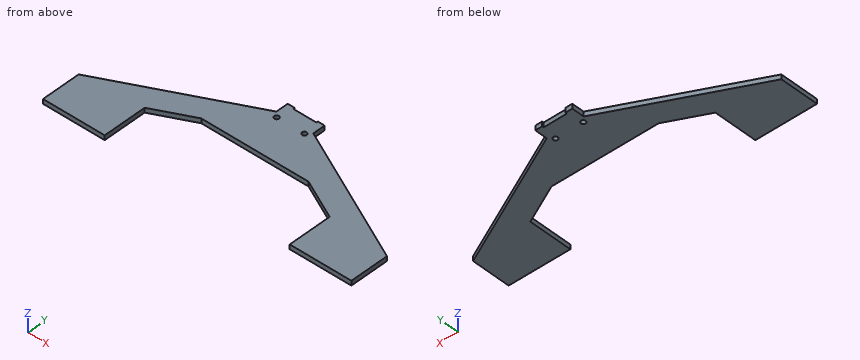
from build123d import *

# Parameters (mm, degrees)
EXTRUDE_1_DEPTH     = 3
SKETCH_3_R          = 1.5
CUT_EXTRUDE_1_DEPTH = 3


with BuildPart() as part:
    # 草图2 → 凸台-拉伸1 (new body)
    with BuildSketch(Plane(origin=(356.17996861, -2895.528235046, -3033.98121825), x_dir=(1, 0, 0), z_dir=(0, 0, 1))):
        Polygon((-296.17996861, 2848.06839364), (-321.386084558, 2860.528235046), (-390.973852662, 2860.528235046), (-416.17996861, 2848.06839364), (-416.17996861, 2820.028235046), (-456.17996861, 2820.028235046), (-456.17996861, 2845.028235046), (-368.17996861, 2888.528235046), (-368.17996861, 2896.528235046), (-363.67996861, 2896.528235046), (-363.67996861, 2895.528235046), (-348.67996861, 2895.528235046), (-348.67996861, 2896.528235046), (-344.17996861, 2896.528235046), (-344.17996861, 2888.528235046), (-256.17996861, 2845.028235046), (-256.17996861, 2820.028235046), (-296.17996861, 2820.028235046), align=None)
    extrude(amount=EXTRUDE_1_DEPTH)

    # 草图3 → 切除-拉伸1 (cut)
    with BuildSketch(Plane.XY.offset(-3030.98121825)):
        with Locations((9, -10)):
            Circle(SKETCH_3_R)
        with Locations((-9, -10)):
            Circle(SKETCH_3_R)
    extrude(amount=-CUT_EXTRUDE_1_DEPTH, mode=Mode.SUBTRACT)


solid = part.part
Input: part model. Units: mm. Frame: model coordinates. Round coordinates to 2 decimals unless told otherwise and drop trailing zeros. Loops run counter-clockwise (first coordinate to the right, second up) from the corner with the lowest first, then second, coordinate; pieces in that order, holes last. Notation, with made-up numbers: (65, -38) -> (84, -38) arc R16 ccw to (84, -11) -> close; hole circle Ø5 at (-23.75, 57). An arc over 180 degrees is marked (long way). Answer as a JSON object with one key per item and string values. Group by question number.
1) Section query D-D on x = -51.5. Output: boundary loops of the cut face in (y, z), plus the area to 3 significant figures.
2) Section query C-C on y = -30. Output: boundary loops of the cut face in (x, z).
3) Section query A-A on z = -3031.7. Output: boundary loops of the cut face in (x, y).
4) Ray query, L1, parallel to X at y = -52, z = -3032.15; L2, parallel to Y at x = -9, z = -3031.8; L3, parallel to Y at x = 5.5, z = -3032.4. Return the intervals inside material, ascending.
5) Pin query (flat end, axial travel): pin 1 (0.9 mm diameter, centred on x = -2.5, z = -3032, fed in from +Y). Return the tip coordinate at first contact, or that it passes through.
6) Section query B-B on y = -69. Output: boundary loops of the cut face in (x, z), plus the area to 3 significant figures.
Reply:
{
 "1": {"outline": "(-43.26, -3033.98) -> (-26.53, -3033.98) -> (-26.53, -3030.98) -> (-43.26, -3030.98) -> close", "area": "50.2 mm2"},
 "2": {"outline": "(-58.53, -3033.98) -> (58.53, -3033.98) -> (58.53, -3030.98) -> (-58.53, -3030.98) -> close"},
 "3": {"outline": "(-100, -75.5) -> (-60, -75.5) -> (-60, -47.46) -> (-34.79, -35) -> (34.79, -35) -> (60, -47.46) -> (60, -75.5) -> (100, -75.5) -> (100, -50.5) -> (12, -7) -> (12, 1) -> (7.5, 1) -> (7.5, 0) -> (-7.5, 0) -> (-7.5, 1) -> (-12, 1) -> (-12, -7) -> (-100, -50.5) -> close; hole circle Ø3 at (-9, -10); hole circle Ø3 at (9, -10)"},
 "4": {"L1": "x = -100 to -60, 60 to 100", "L2": "y = -35 to -11.5, -8.5 to 1", "L3": "y = -35 to 0"},
 "5": {"pin 1": "stops at y = 0"},
 "6": {"outline": "(-100, -3033.98) -> (-60, -3033.98) -> (-60, -3030.98) -> (-100, -3030.98) -> close; (60, -3033.98) -> (100, -3033.98) -> (100, -3030.98) -> (60, -3030.98) -> close", "area": "240 mm2"}
}
